from build123d import *

# Parameters (mm, degrees)
BOSS_EXTRUDE1_DEPTH = 30.69
BOSS_EXTRUDE2_DEPTH = 8
BOSS_EXTRUDE3_DEPTH = 40.11
BOSS_EXTRUDE4_DEPTH = 3.48


with BuildPart() as part:
    # Sketch3 → Boss-Extrude1 (new body)
    with BuildSketch(Plane(origin=(0, 0, 0), x_dir=(1, 0, 0), z_dir=(0, 1, 0))):
        with BuildLine():
            ThreePointArc((-5.048331501, 1.771115202), (-4.364514081, -3.094110023), (0, -5.35))
            Line((0, -5.35), (0, -4.57))
            ThreePointArc((0, -4.57), (-4.57, 0), (0, 4.57))
            Line((0, 4.57), (0, 5.35))
            ThreePointArc((0, 5.35), (-3.094110023, 4.364514081), (-5.048331501, 1.771115202))
        make_face()
        with BuildLine():
            Line((0, -4.57), (0, -5.35))
            ThreePointArc((0, -5.35), (3.783021279, -3.783021279), (5.35, 0))
            ThreePointArc((5.35, 0), (5.274043682, 0.898311324), (5.048331501, 1.771115202))
            ThreePointArc((5.048331501, 1.771115202), (3.094110023, 4.364514081), (0, 5.35))
            Line((0, 5.35), (0, 4.57))
            ThreePointArc((0, 4.57), (3.23147799, 3.23147799), (4.57, 0))
            ThreePointArc((4.57, 0), (3.23147799, -3.23147799), (0, -4.57))
        make_face()
    extrude(amount=BOSS_EXTRUDE1_DEPTH)

    # Sketch3_5 → Boss-Extrude2 (add)
    with BuildSketch(Plane(origin=(0, 0, 0), x_dir=(1, 0, 0), z_dir=(0, 1, 0))):
        with BuildLine():
            Line((0, 8.65), (0, 5.35))
            ThreePointArc((0, 5.35), (3.094110023, 4.364514081), (5.048331501, 1.771115202))
            Line((5.048331501, 1.771115202), (2.635, 8.65))
            Line((2.635, 8.65), (0, 8.65))
        make_face()
        with BuildLine():
            Line((-2.635, 8.65), (-5.048331501, 1.771115202))
            ThreePointArc((-5.048331501, 1.771115202), (-3.094110023, 4.364514081), (0, 5.35))
            Line((0, 5.35), (0, 8.65))
            Line((0, 8.65), (-2.635, 8.65))
        make_face()
    extrude(amount=BOSS_EXTRUDE2_DEPTH)

    # Sketch5 → Boss-Extrude3 (add)
    with BuildSketch(Plane(origin=(0, 8, 0), x_dir=(1, 0, 0), z_dir=(0, 1, 0))):
        Polygon((-3.30158041, 6.75), (3.30158041, 6.75), (2.635, 8.65), (-2.635, 8.65), align=None)
    extrude(amount=BOSS_EXTRUDE3_DEPTH)

    # Sketch3_6 → Boss-Extrude4 (add)
    with BuildSketch(Plane(origin=(0, 0, 0), x_dir=(1, 0, 0), z_dir=(0, 1, 0))):
        with BuildLine():
            ThreePointArc((0, 4.57), (-4.57, 0), (0, -4.57))
            Line((0, -4.57), (0, 4.57))
        make_face()
        with BuildLine():
            Line((0, 4.57), (0, -4.57))
            ThreePointArc((0, -4.57), (3.23147799, -3.23147799), (4.57, 0))
            ThreePointArc((4.57, 0), (3.23147799, 3.23147799), (0, 4.57))
        make_face()
    extrude(amount=BOSS_EXTRUDE4_DEPTH)


solid = part.part
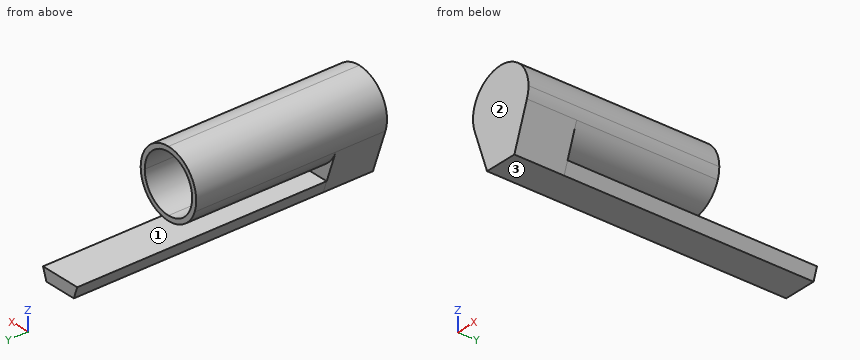
Geometry check sheet. Reference: the model listing, model coordinates, mm. Face numbers are marked on the shaded views. Round coordinates to 2 decimals unless told otherwise and drop trailing zeros. Order: outer loops, then holes, each group sorted by start corner. A loop starts at its lowest first (then second) coordinate and runs counter-clockwise, first axis right, second up. Notation, with made-up numbers: M 68,-7.5 L 117,-7.5 A37 ccw 117,28.5 Z; hole C -26,-29.75 d8. An arc over 180 degrees is marked long. Answer in a Markdown table with one row per item.
(1) Sectioned sample at C-C, the plane x = -2. Record the cut outline in (y, z), and give its area (3 significant figures).
Responses:
| item | result |
|---|---|
| outline | M 0,-8.65 L 48.11,-8.65 L 48.11,-6.75 L 8,-6.75 L 8,-4.96 L 30.69,-4.96 L 30.69,-4.11 L 3.48,-4.11 L 3.48,4.11 L 30.69,4.11 L 30.69,4.96 L 0,4.96 Z |
| area | 187 mm² |
(2) Draft check along Z on the marked faces 1, 2 and 3. Enter one of: released by +Z, released by -Z, zero draft, split by the parting line, or undercut.
Responses:
| item | result |
|---|---|
| face 1 | undercut |
| face 2 | zero draft |
| face 3 | released by -Z |
(3) Go/stop test with flat-tipped pins: P1, Ø3, axis at x = -4, y = 6, coming from the +Z side; P2, Ø4, axis at x = -0.5, z = -3, coming from the +Y side; P3, Ø1, axis at x = -2.5, y = 21.5, coming from the +Z side; P4, Ø3.5, axis at x = -1.5, y = 20, coming from the +Z side. Record where each tip stops, or that it passes through.
Responses:
| item | result |
|---|---|
| P1 | stops at z = 4.73 |
| P2 | stops at y = 30.69 |
| P3 | stops at z = 4.96 |
| P4 | stops at z = 5.35 |
(4) Sectioned sample at D-D, the plane y = 39. Record the cut outline in (x, z) (3 decimals), and give its area (3 significant figures).
Responses:
| item | result |
|---|---|
| outline | M -3.302,-6.75 L -2.635,-8.65 L 2.635,-8.65 L 3.302,-6.75 Z |
| area | 11.3 mm² |
(5) Sectioned sample at A-A, the plane y = 21.5. Record the cut outline in (x, z) (3 decimals).
Responses:
| item | result |
|---|---|
| outline | C 0,0 d10.7; M -3.302,-6.75 L -2.635,-8.65 L 2.635,-8.65 L 3.302,-6.75 Z; hole C 0,0 d9.14 |
(6) Scan lines: probe 1 along Z at (x, y) = (-0.25, 12.5); probe 2 along X at (y, z) = (7.5, -0.25); probe 3 along Z at (x, y) = (-1, 25.5). Record each from-to range of solid material in increasing order. Write a range as from..to.
Responses:
| item | result |
|---|---|
| probe 1 | z = -8.65..-6.75, -5.34..-4.56, 4.56..5.34 |
| probe 2 | x = -5.34..-4.56, 4.56..5.34 |
| probe 3 | z = -8.65..-6.75, -5.26..-4.46, 4.46..5.26 |
(7) Sectioned sample at B-B, the plane z = 2.75. Record the cut outline in (x, y), and give its area (3 significant figures).
Responses:
| item | result |
|---|---|
| outline | M -4.59,0 L 4.59,0 L 4.59,30.69 L 3.65,30.69 L 3.65,3.48 L -3.65,3.48 L -3.65,30.69 L -4.59,30.69 Z |
| area | 83.0 mm² |
